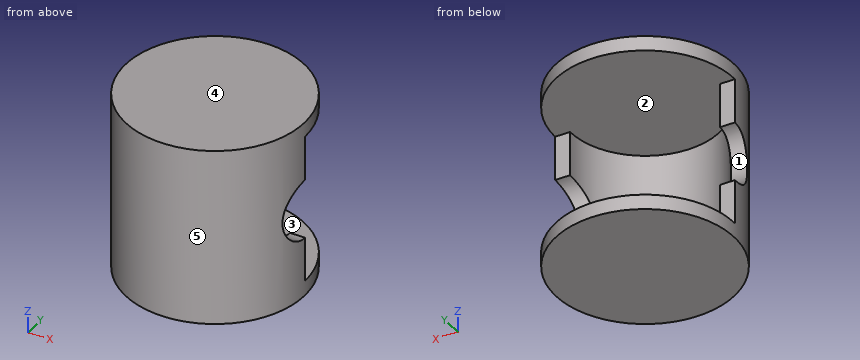
```python
from build123d import *

# Parameters (mm, degrees)
F0_R     = 76.2
F1_DEPTH = 152.4
F2_W     = 76.771498
F2_H     = 127
F3_DEPTH = 76.2
F4_R     = 63.5
F5_DEPTH = 127
F6_R     = 25.4
F7_DEPTH = 76.2


with BuildPart() as f1:
    # F0 (on Top) → F1 (new body)
    with BuildSketch(Plane.XY):
        Circle(F0_R)
    extrude(amount=F1_DEPTH)

    # F2 (on Right) → F3 (cut, symmetric)
    with BuildSketch(Plane.YZ):
        with Locations((38.385749, 76.2)):
            Rectangle(F2_W, F2_H)
    extrude(amount=F3_DEPTH, both=True, mode=Mode.SUBTRACT)

    # F4 (on face) → F5 (cut)
    with BuildSketch(Plane.XY.offset(12.7)):
        Circle(F4_R)
    extrude(amount=F5_DEPTH, mode=Mode.SUBTRACT)

    # F6 (on Right) → F7 (cut, symmetric)
    with BuildSketch(Plane.YZ):
        with Locations((0, 76.2)):
            Circle(F6_R)
    extrude(amount=F7_DEPTH, both=True, mode=Mode.SUBTRACT)


solid = f1.part
```
Design review of the part built by this model. Coordinates are the model's own, in mm. Face numbers are marked on the shaded views. A direction names the side the tool comes from. Give positions to 0.01 mm unless a question says otherwise; leave off trailing zeros. Order: outer loops, then holes, each group sorted by start corner. A loop starts at its lowest first (then second) coordinate and runs counter-clockwise, first axis right, second up. Notation, with made-up numbers: (-12.75, -31.5) - (-2.75, -31.5) arc R10 ccw to (-2.75, -15.5) - close; hole circle Ø7 at (-5.5, 72.5). An arc over 180 degrees is marked (long way). Use a Markdown table: item, result. Add a question column.
(1) Add section A-A on y = 12.5. Give the boundary of the cut face in (x, z), then the cut area to 3 significant figures.
(2) Add section D-D on z = 45. Give the boundary of the cut face in (x, y).
(3) Machinability: for the marked faces 1 and 2, which of the approach directions +Z, -Z, +X, -X, +Y, -Y give a long, thin tool a straight path to every point of the face, cutting with its end or side? Answer none if there is none.
(4) Add section C-C on y = -38.5. Give the boundary of the cut face in (x, z), then the cut area to 3 significant figures.
(5) Add section B-B on x = 0. Give the boundary of the cut face in (y, z).
(6) Mouldability with a two-part tool opening along X and no side actions: class the marked faces 3, 4 and 5 as +X half, -X half, draft (parallel to the pull), parting line (faces both ways), or undercut.
(7) Clearance check with flat-ended pins moving along their axes: P1, Ø5, axis at x = 47, z = 36, coming from the -Y side; P2, Ø4, axis at x = -69, z = 113.5, coming from the +Y side; P3, Ø2, axis at y = -32, z = 88, coming from the -X side. State where each tip first meets the part, or that it passes through.
(8) Wall thickness on probe 1 along Z at (x, y) = (-7, 51); probe 2 along X at (y, z) = (-43, 87.5); probe 3 along X at (y, z) = (-46.5, 126.5): over which ranges is each line inside the solid? List them lowest first. Write a range as [from, to].
Report:
| question | item | result |
|---|---|---|
| 1 | outline | (-75.17, 0) - (75.17, 0) - (75.17, 12.7) - (-75.17, 12.7) - close; (-75.17, 139.7) - (75.17, 139.7) - (75.17, 152.4) - (-75.17, 152.4) - close |
| 1 | area | 3,820 mm² |
| 2 | outline | (-76.2, 0) arc R76.2 ccw to (76.2, 0) - (63.5, 0) arc R63.5 cw to (-63.5, 0) - close |
| 3 | face 1 | +X, -X, +Y |
| 3 | face 2 | +Y |
| 4 | outline | (-65.76, 0) - (65.76, 0) - (65.76, 152.4) - (-65.76, 152.4) - close; hole (-50.5, 12.7) - (50.5, 12.7) - (50.5, 139.7) - (-50.5, 139.7) - close |
| 4 | area | 7,220 mm² |
| 5 | outline | (-76.2, 0) - (76.2, 0) - (76.2, 12.7) - (-63.5, 12.7) - (-63.5, 139.7) - (76.2, 139.7) - (76.2, 152.4) - (-76.2, 152.4) - close |
| 6 | face 3 | undercut |
| 6 | face 4 | draft |
| 6 | face 5 | parting line |
| 7 | P1 | stops at y = -61.86 |
| 7 | P2 | stops at y = 0 |
| 7 | P3 | stops at x = -69.61 |
| 8 | probe 1 | z = [0, 12.7], [139.7, 152.4] |
| 8 | probe 2 | x = [-62.91, -46.73], [46.73, 62.91] |
| 8 | probe 3 | x = [-60.37, -43.24], [43.24, 60.37] |
